```python
from build123d import *

# Parameters (mm, degrees)
F0_R     = 12.49
F1_DEPTH = 2.84
F2_R     = 10.74
F3_DEPTH = 0.12
F4_R     = 11.08
F5_DEPTH = 26.56
F6_R     = 6.4
F7_DEPTH = 29.52
F8_R     = 0.5


with BuildPart() as f1:
    # F0 (on Right) → F1 (new body)
    with BuildSketch(Plane.YZ):
        Circle(F0_R)
    extrude(amount=F1_DEPTH)

    # F2 (on face) → F3 (join)
    with BuildSketch(Plane.YZ.offset(2.84)):
        Circle(F2_R)
    extrude(amount=F3_DEPTH)

    # F4 (on face) → F5 (join)
    with BuildSketch(Plane.YZ.offset(2.96)):
        Circle(F4_R)
    extrude(amount=F5_DEPTH)

    # F6 (on face) → F7 (cut)
    with BuildSketch(Plane(origin=(0, 0, 0), x_dir=(0, -1, 0), z_dir=(-1, 0, 0))):
        Circle(F6_R)
    extrude(amount=-F7_DEPTH, mode=Mode.SUBTRACT)

    # F8
    f8_edges = [f1.edges().sort_by_distance(p)[0] for p in [
        (0, 6.4, 0),
        (29.52, -11.08, 0),
        (29.52, 6.4, 0),
    ]]
    fillet(f8_edges, radius=F8_R)


solid = f1.part
```
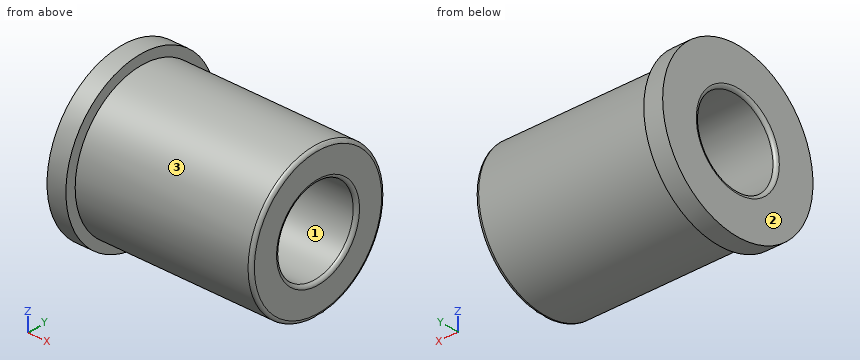
Can you work these out from the model? Positions are in its coordinate system, mm. Face numbers are marked on the shaded views. Round coordinates to 2 decimals unless told otherwise and drop trailing zeros. Loops run counter-clockwise (first coordinate to the right, second up) from the corner with the lowest first, then second, coordinate; pieces in that order, holes last. Notation, with made-up numbers: M 65.5,42 L 94.5,42 A35 ccw 94.5,75 Z; hole C -8,27.25 d3. An arc over 180 degrees is marked long. Answer as a JSON object with one key per item and string values. Group by question number.
Q1. We'd pull the mould along Y, two halves only. Please class the marked faces 1, 2 and 3: +Y half, -Y half, draft (parallel to the pull), parting line (faces both ways), or undercut.
Q2. Imagine slicing it at B-B, the plane x = 6.75. Please give me the cut outline in (y, z), then the cut area to 3 significant figures.
Q3. Will these pins go through, and if not, where does the flat tip stop? pin 1 (8 mm diameter, centred on y = 5.5, z = 1, fed in from -X); pin 2 (6 mm diameter, centred on x = 18.5, z = 7, fed in from -Y); pin 3 (4 mm diameter, centred on x = 19.5, z = 5.5, fed in from -Y); pin 4 (1 mm diameter, centred on x = 20.5, z = -6, fed in from -Y).
Q4. Please list where these lines run through material, in increasing order: L1, parallel to Z at x = 13, y = 0; L2, parallel to X at y = 10.5, z = -1.75; L3, parallel to Z at x = 5.25, y = -4.5.
Q5. Imagine slicing it at A-A, the plane y = 0. Please give me the cut outline in (x, z).
Findings:
{
 "1": {"face 1": "undercut", "face 2": "draft", "face 3": "parting line"},
 "2": {"outline": "C 0,0 d22.16; hole C 0,0 d12.8", "area": "257 mm2"},
 "3": {"pin 1": "stops at x = 0", "pin 2": "stops at y = -10.33", "pin 3": "stops at y = -10.51", "pin 4": "stops at y = -9.62"},
 "4": {"L1": "z = -11.08 to -6.4, 6.4 to 11.08", "L2": "x = 0 to 29.52", "L3": "z = -10.13 to -4.55, 4.55 to 10.13"},
 "5": {"outline": "M 0,-12.49 L 2.84,-12.49 L 2.84,-10.74 L 2.96,-10.74 L 2.96,-11.08 L 29.02,-11.08 A0.5 ccw 29.52,-10.58 L 29.52,-6.9 A0.5 ccw 29.02,-6.4 L 0.5,-6.4 A0.5 ccw 0,-6.9 Z; M 0,6.9 A0.5 ccw 0.5,6.4 L 29.02,6.4 A0.5 ccw 29.52,6.9 L 29.52,10.58 A0.5 ccw 29.02,11.08 L 2.96,11.08 L 2.96,10.74 L 2.84,10.74 L 2.84,12.49 L 0,12.49 Z"}
}
